from build123d import *

# Parameters (mm, degrees)
SKETCH2_R           = 12.7
SKETCH2_R_2         = 9.2837
BOSS_EXTRUDE1_DEPTH = 2.54
SKETCH3_R           = 9.525
SKETCH3_R_2         = 6.858
BOSS_EXTRUDE2_DEPTH = 2.54
FILLET1_R           = 0.2032
CHAMFER1_SIZE       = 0.254


with BuildPart() as part:
    # Sketch2 → Boss-Extrude1 (new body)
    with BuildSketch(Plane(origin=(0, 0, 0), x_dir=(1, 0, 0), z_dir=(0, 1, 0))):
        with Locations(Location((0, 0, 0), (0, 0, 270))):
            Circle(SKETCH2_R)
        with Locations(Location((0, 0, 0), (0, 0, 270))):
            Circle(SKETCH2_R_2, mode=Mode.SUBTRACT)
    extrude(amount=BOSS_EXTRUDE1_DEPTH)

    # Sketch3 → Boss-Extrude2 (add)
    with BuildSketch(Plane(origin=(0, 2.54, 0), x_dir=(1, 0, 0), z_dir=(0, 1, 0))):
        with Locations(Location((0, 0, 0), (0, 0, 270))):
            Circle(SKETCH3_R)
        with Locations(Location((0, 0, 0), (0, 0, 270))):
            Circle(SKETCH3_R_2, mode=Mode.SUBTRACT)
    extrude(amount=BOSS_EXTRUDE2_DEPTH)

    # Fillet1
    fillet1_edges = [part.edges().sort_by_distance(p)[0] for p in [
        (0, 2.54, -9.2837),
        (0, 2.54, -9.525),
    ]]
    fillet(fillet1_edges, radius=FILLET1_R)

    # Chamfer1
    chamfer1_edges = [part.edges().sort_by_distance(p)[0] for p in [
        (0, 5.08, -6.858),
        (0, 2.54, -12.7),
        (0, 0, -12.7),
        (0, 0, -9.2837),
        (0, 5.08, -9.525),
    ]]
    chamfer(chamfer1_edges, length=CHAMFER1_SIZE)


solid = part.part
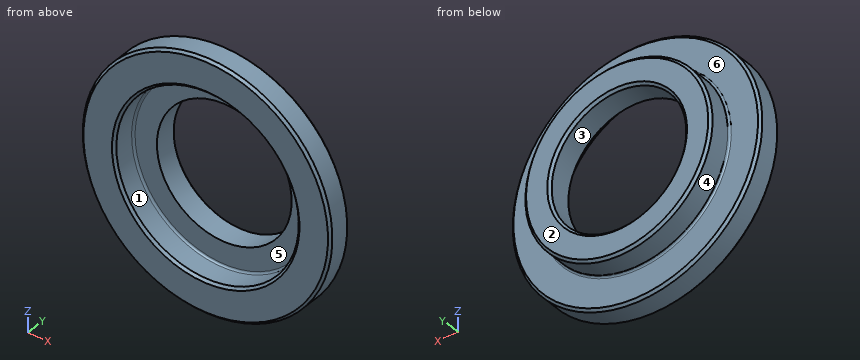
Can you work these out from the model? Positions are in its coordinate system, mm. Face numbers are marked on the shaded views. A direction names the side the tool comes from. Round coordinates to 2 decimals unless told otherwise and drop trailing zeros. Write each loop counter-clockwise with the first axis right and the second up, starting at its lowest first coordinate (ties: lowest second). Pieces come first, ordered by that corner, then holes. Notation, with made-up numbers: M -5,82 L 35,82 A17 cw 35,98 Z; hole C 60,10.25 d11. An arc over 180 degrees is marked long. Use a Markdown table: item, result.
Item 1: I want a section at C-C (y = 1.7). List the corners of the cut face in (x, z) for me, and give its area (3 significant figures).
Found:
| item | result |
|---|---|
| outline | C 0,0 d25.4; hole C 0,0 d18.57 |
| area | 236 mm2 |
Item 2: We'd pull the mould along Z, two halves only. Please class the marked faces 3, 4, 5 and 6: released by +Z, released by -Z, zero draft, split by the parting line, or undercut.
Found:
| item | result |
|---|---|
| face 3 | undercut |
| face 4 | split by the parting line |
| face 5 | undercut |
| face 6 | zero draft |
Item 3: Which directions (+Z, -Z, +X, -X, +Y, -Y) give clear straight access to the entire face, cutting with the end or side of a thin tool? Please do the marked faces 1 and 2.
Found:
| item | result |
|---|---|
| face 1 | -Y |
| face 2 | +Z, -Z, +X, -X, +Y |
Item 4: I want a section at D-D (y = 4.4). List the corners of the cut face in (x, z) for me (3 decimals), and give its area (3 significant figures).
Found:
| item | result |
|---|---|
| outline | C 0,0 d19.05; hole C 0,0 d13.716 |
| area | 137 mm2 |
Item 5: For pin 1 Ø2 at (x, z) = (5.5, 4) entering from -Y, with a flat end and sliding along its axis, tell me the tip position at first contact or that it passes through.
Found:
| item | result |
|---|---|
| pin 1 | stops at y = 2.54 |
Item 6: If I drill on line 1 along X through (y, z) = (4.25, 0) (3 decimals); line 2 along X through (y, z) = (1.1, 0); line 3 along Z through (x, y) = (0.25, 3.5), over which ranges is the centre line in solid material (lowest first)? Write a range as [from, to].
Found:
| item | result |
|---|---|
| line 1 | x = [-9.525, -6.858], [6.858, 9.525] |
| line 2 | x = [-12.7, -9.28], [9.28, 12.7] |
| line 3 | z = [-9.52, -6.85], [6.85, 9.52] |
